Design review of the part shown in the three views and the two pictorial views. Dimensions are in mm from the part's minimum x, y and z. A direction names the side the tool comes from. Coordinates: 2 decimals unless noted, no trailing zeros. Loops run counter-clockwise (first coordinate to the right, second up) from the corner with the lowest first, then second, coordinate; pieces in that order, holes last. Notation, with made-up numbers: (60.5, 84) - (65.5, 84) arc R14 cw to (65.5, 94) - close; hole circle Ø1 at (60, 16.5). An arc over 180 degrees is marked (long way). One line per question, with ' | ' between items.
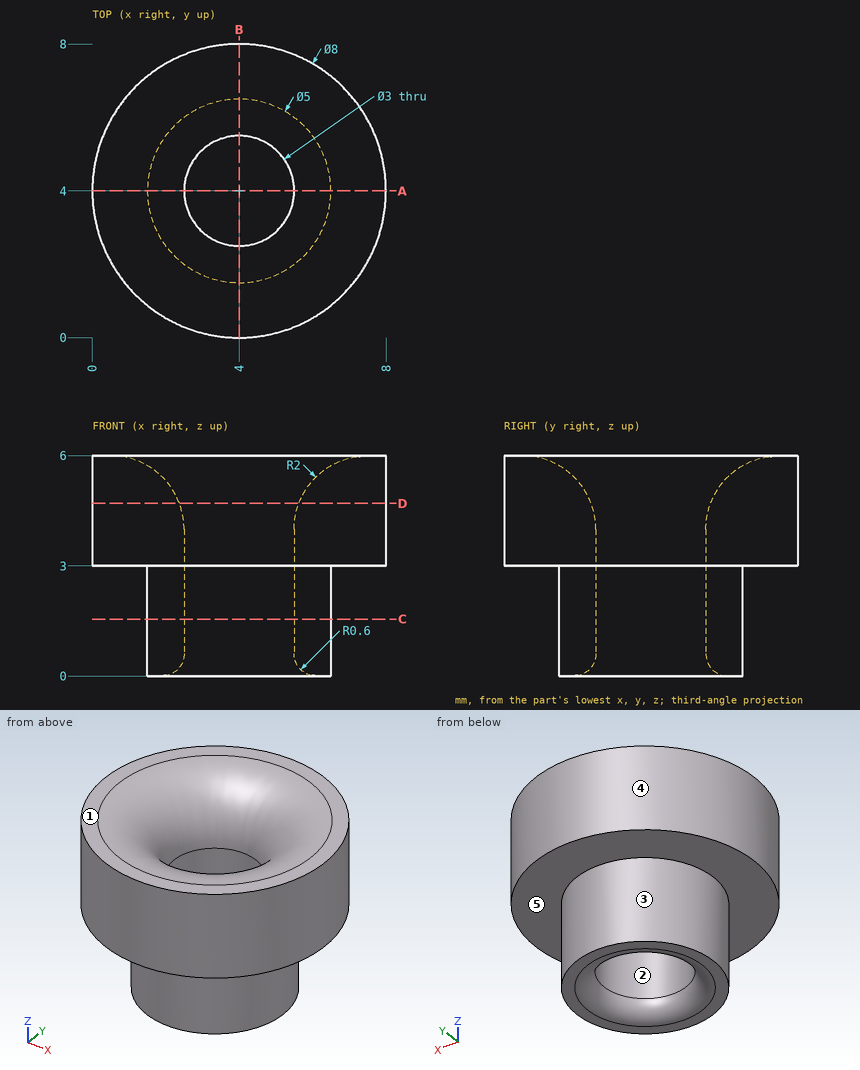
Q1. Tool access review of the marked faces 4 and 5: name each direction out of +Z, -Z, +X, -X, +Y, -Y from which nothing blocks a thin tool from reaching the whole face with its end or side.
Returned:
face 4: +Z, -Z | face 5: -Z
Q2. For pin 1 (1.5 mm diameter, centred on x = 5.5, z = 1, fed in from -Y); pin 2 (2.5 mm diameter, centred on x = 3.5, y = 2.5, fed in from -Z); pin 3 (3.5 mm diameter, centred on x = 4, y = 4, fed in from +Z); pin 4 (1.5 mm diameter, centred on y = 5.5, z = 2.5, fed in from -X), all flat-tipped, find the tip position at first contact; note any pin that passes through.
Returned:
pin 1: stops at y = 1.62 | pin 2: stops at z = 0 | pin 3: stops at z = 4.97 | pin 4: stops at x = 0.11
Q3. Take a section at C-C (z = 1.55). Give the boundary of the cut face in (x, y), plus the area to 3 significant figures.
Returned:
outline: circle Ø5 at (4, 4); hole circle Ø3 at (4, 4) | area: 12.6 mm²
Q4. Take a section at A-A (y = 4). Give the boundary of the cut face in (x, z), plus the area to 3 significant figures.
Returned:
outline: (0, 3) - (1.5, 3) - (1.5, 0) - (1.9, 0) arc R0.6 ccw to (2.5, 0.6) - (2.5, 4) arc R2 ccw to (0.5, 6) - (0, 6) - close; (5.5, 0.6) arc R0.6 ccw to (6.1, 0) - (6.5, 0) - (6.5, 3) - (8, 3) - (8, 6) - (7.5, 6) arc R2 ccw to (5.5, 4) - close | area: 19.1 mm²
Q5. Take a section at D-D (z = 4.7). Give the boundary of the cut face in (x, y).
Returned:
outline: circle Ø8 at (4, 4); hole circle Ø3.25 at (4, 4)
Q6. Draft analysis for pull direction X (two halves, no side actions). For the marked faces 1, 2 and 3, state which applies: +X half, -X half, draft (parallel to the pull), parting line (faces both ways), or undercut.
Returned:
face 1: draft | face 2: undercut | face 3: parting line
Q7. To check wall thickness, follow line 1 along Y through (x, z) = (4, 2.15); line 2 along Y through (x, z) = (4, 3.3); line 3 along X through (y, z) = (3, 0.75). State the ranges of each line that lie inside material, in increasing order.
Returned:
line 1: y = 1.5 to 2.5, 5.5 to 6.5 | line 2: y = 0 to 2.5, 5.5 to 8 | line 3: x = 1.71 to 2.88, 5.12 to 6.29
